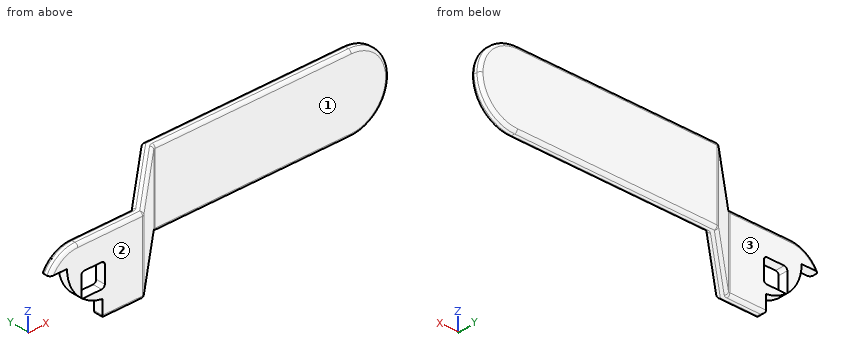
from build123d import *

# Parameters (mm, degrees)
EXTRUDE_THIN1_DEPTH = 24
CUT_EXTRUDE1_DEPTH  = 131.847239176
FILLET1_R           = 10
FILLET2_R           = 12
FILLET3_R           = 1
FILLET4_R           = 1


# Some blends are built 0.0001 mm under size
with BuildPart() as part:
    # Sketch1 → Extrude-Thin1 (new body)
    with BuildSketch(Plane.XY):
        Polygon((0, 0), (30, 0), (52, 20.396078054), (127, 20.396078054), (127, 23.396078054), (50.823303189, 23.396078054), (28.823303189, 3), (0, 3), align=None)
    extrude(amount=-EXTRUDE_THIN1_DEPTH)

    # Sketch2 → Cut-Extrude1 (cut, through all)
    with BuildSketch(Plane(origin=(0, 3, 0), x_dir=(1, 0, 0), z_dir=(0, 1, 0))):
        with BuildLine():
            Line((16.823303189, 24), (0, 24))
            Line((0, 24), (0, 5.5))
            Line((0, 5.5), (5.5, 5.5))
            ThreePointArc((5.5, 5.5), (6.698004209, 10.97816866), (10.073303189, 15.456215417))
            Line((10.073303189, 15.456215417), (10.073303189, 8.25))
            Line((10.073303189, 8.25), (17.573303189, 8.25))
            Line((17.573303189, 8.25), (17.573303189, 15.75))
            Line((17.573303189, 15.75), (10.427766753, 15.75))
            ThreePointArc((10.427766753, 15.75), (13.439867838, 17.556796696), (16.823303189, 18.5))
            Line((16.823303189, 18.5), (16.823303189, 24))
        make_face()
    extrude(amount=-CUT_EXTRUDE1_DEPTH, mode=Mode.SUBTRACT)

    # Fillet1
    # the kernel refuses this fillet: 10 mm, written as the material it takes off along each edge
    with BuildSketch(Plane(origin=(0, 25.325713874, 0), x_dir=(1, 0, 0), z_dir=(0, -1, 0))) as fillet1_piece_1:
        with BuildLine():
            CenterArc((8.93028555, -10), FILLET1_R, 90, 63.25631605)
            Line((0, -5.5), (-0.178605711, -5.41))
            ThreePointArc((-0.178605711, -5.41), (-0.2, -2.75), (-0.2, 0))
            Line((-0.2, 0), (0, 0.2))
            Line((0, 0.2), (8.93028555, 0.2))
            Line((8.93028555, 0.2), (8.93028555, 0))
        make_face()
    extrude(amount=47.651427749, mode=Mode.SUBTRACT)

    # Fillet2
    fillet2_edges = [part.edges().sort_by_distance(p)[0] for p in [
        (127, 21.896078054, 0),
        (127, 21.896078054, -24),
    ]]
    fillet(fillet2_edges, radius=FILLET2_R - 0.0001)  # a hair under: the kernel refuses the full size

    # Fillet3
    fillet3_edges = [part.edges().sort_by_distance(p)[0] for p in [
        (52, 20.396078054, -12),
        (30, 0, -12),
        (28.823303189, 3, -12),
        (50.823303189, 23.396078054, -12),
        (82.911701595, 23.396078054, -24),
        (39.823303189, 13.198039027, -24),
        (23.411651595, 0, -24),
        (22.823303189, 3, -24),
        (16.823303189, 1.5, -24),
        (41, 10.198039027, -24),
        (83.50005, 20.396078054, -24),
        (18.876794369, 3, 0),
        (3.686241309, 3, -1.485306817),
        (19.465142775, 0, 0),
        (3.686241309, 0, -1.485306817),
        (123.485310664, 20.396078054, -20.485310664),
        (123.485310664, 20.396078054, -3.514689336),
        (123.485310664, 23.396078054, -20.485310664),
        (123.485310664, 23.396078054, -3.514689336),
        (41, 10.198039027, 0),
        (39.823303189, 13.198039027, 0),
        (82.911701595, 23.396078054, 0),
        (83.50005, 20.396078054, 0),
    ]]
    fillet(fillet3_edges, radius=FILLET3_R)

    # Fillet4
    fillet4_edges = [part.edges().sort_by_distance(p)[0] for p in [
        (17.573303189, 1.5, -15.75),
        (17.573303189, 1.5, -8.25),
        (10.073303189, 1.5, -8.25),
    ]]
    fillet(fillet4_edges, radius=FILLET4_R)


solid = part.part
Here's how the part is built. I have some questions about the finished solid (model axes, mm). Face numbers are marked on the shaded views. A direction names the side the tool comes from. Round coordinates to 2 decimals unless told otherwise and drop trailing zeros. Write each loop counter-clockwise with the first axis right and the second up, starting at its lowest first coordinate (ties: lowest second). Pieces come first, ordered by that corner, then holes.
1. For the marked faces 1, 2 and 3, which set-ups out of +Z, -Z, +X, -X, +Y, -Y let a thin tool reach every point of the face, with its end or its side?
2. I need wall thicknesses on L1, parallel to Y at x = 26.5, z = -3; L2, parallel to Y at x = 97, z = -18.5; L3, parallel to X at y = 3.25, z = -11.25. Which ranges of each line are inside material? Lowest first, please.
3. Suppose I cut it at A-A (x = 63). List the corners of the cut face in (y, z) for me.
4. Will these pins go through, and if not, where does the flat tip stop? pin 1 Ø6 at (x, y) = (63, 18.5) entering from +Z; pin 2 Ø1.5 at (y, z) = (1.5, -12.5) entering from +X; pin 3 Ø3.5 at (x, y) = (14, 1) entering from -Z; pin 4 Ø1 at (x, z) = (93, -12.5) entering from -Y.
Answer sheet:
1. face 1: +Z, -Z, +X, -Y
1. face 2: +Z, -Z, +X, -X, -Y
1. face 3: +Z, -Z, -X, +Y
2. L1: y = 0 to 3
2. L2: y = 20.4 to 23.4
2. L3: x = 29.09 to 33.51
3. outline: (20.4, -23) arc R1 ccw to (21.4, -24) - (22.4, -24) arc R1 ccw to (23.4, -23) - (23.4, -1) arc R1 ccw to (22.4, 0) - (21.4, 0) arc R1 ccw to (20.4, -1) - close
4. pin 1: stops at z = 0
4. pin 2: stops at x = 32.43
4. pin 3: stops at z = -18.31
4. pin 4: stops at y = 20.4
